Input: part model. Units: mm. Frame: model coordinates. A direction names the side the tool comes from. Coordinates: 2 decimals unless noted, no trailing zeros. Write each loop counter-clockwise with the first axis right and the second up, starting at its lowest first coordinate (ties: lowest second). Pieces come first, ordered by that corner, then holes. Notation, with made-up numbers: M 72,-38 L 83,-38 A8 cw 83,-26 Z; hole C -40,63 d10. An arc over 180 degrees is marked long. Write each question's results on one line, items separated by ' | '. Start each with the question number.
1. Set-up query: faces 1 (the flat face through (188, -110, 9)), 2 (the flat face through (104, -118, 11)). Return all of +Z, -Z, +X, -X, +Y, -Y with unobstructed straight access to the full face (end or side cutting, diameter ignored); none if empty.
2. First-contact query: pin 1 (5.5 mm diameter, centred on x = 80, y = -38, fed in from +Z); pin 2 (5 mm diameter, centred on x = 7, y = -6.5, fed in from +Z). Flat tips, straight axial feed; report the tip coordinate or a pass-through.
3. Section query B-B, the plane x = 88. Output: boundary loops of the cut face in (y, z).
4. Pull-direction query (X, two-part tool) for faces 3 (the flat face through (104, -58, 0)), 4 (the flat face through (8, -13, 9)), 5 (the flat face through (210, -60, 11)), 6 (the flat face through (8, -105, 9)); classes: +X half, -X half, draft (parallel to the pull), parting line (faces both ways), or undercut.
5. Section query A-A, the plane z = 5.5. Output: boundary loops of the cut face in (x, y), and give its area (3 significant figures).
6. Section query C-C, the plane y = -89. Output: boundary loops of the cut face in (x, z), and give its area (3 significant figures).
7. Ray query, probe 1 along X at (y, z) = (-110.5, 13); probe 2 along Y at (x, z) = (80, 1.95); probe 3 along X at (y, z) = (-13.5, 18.25). Return the intervals inside material, ascending.
```python
from build123d import *

# Parameters (mm, degrees)
F0_W     = 210
F0_H     = 118
F1_DEPTH = 23
F2_T     = -3
F3_W     = 10
F3_H     = 10
F4_DEPTH = 13
F5_R     = 1.75
F6_DEPTH = 25


with BuildPart() as f1:
    # F0 (on Top) → F1 (new body)
    with BuildSketch(Plane.XY):
        with Locations((105, -59)):
            Rectangle(F0_W, F0_H)
    extrude(amount=F1_DEPTH)

    # F2
    f2_openings = [f1.faces().sort_by_distance(p)[0] for p in [
        (105, -59, 23),
    ]]
    offset(amount=F2_T, openings=f2_openings)

    # F3 (on face) → F4 (join)
    with BuildSketch(Plane.XY.offset(3)):
        with Locations((8, -8)):
            Rectangle(F3_W, F3_H)
        with Locations((183, -8)):
            Rectangle(F3_W, F3_H)
        with Locations((183, -110)):
            Rectangle(F3_W, F3_H)
        with Locations((8, -110)):
            Rectangle(F3_W, F3_H)
    extrude(amount=F4_DEPTH)

    # F5 (on face) → F6 (cut)
    with BuildSketch(Plane.XY.offset(3)):
        with Locations((20, -8)):
            Circle(F5_R)
        with Locations((20, -38)):
            Circle(F5_R)
        with Locations((80, -38)):
            Circle(F5_R)
        with Locations((80, -8)):
            Circle(F5_R)
        with Locations((120, -17.5)):
            Circle(F5_R)
    extrude(amount=-F6_DEPTH, mode=Mode.SUBTRACT)


solid = f1.part
```
Answer:
1) face 1: +Z | face 2: +Z, -Z, +X, -X, -Y
2) pin 1: z = 3 | pin 2: z = 16
3) outline: M -118,0 L 0,0 L 0,23 L -3,23 L -3,3 L -115,3 L -115,23 L -118,23 Z
4) face 3: draft | face 4: undercut | face 5: +X half | face 6: undercut
5) outline: M 0,-118 L 210,-118 L 210,0 L 0,0 Z; hole M 3,-105 L 13,-105 L 13,-115 L 178,-115 L 178,-105 L 188,-105 L 188,-115 L 207,-115 L 207,-3 L 188,-3 L 188,-13 L 178,-13 L 178,-3 L 13,-3 L 13,-13 L 3,-13 Z | area: 2,330 mm^2
6) outline: M 0,0 L 210,0 L 210,23 L 207,23 L 207,3 L 3,3 L 3,23 L 0,23 Z | area: 750 mm^2
7) probe 1: 0 to 13, 178 to 188, 207 to 210 | probe 2: -118 to -39.75, -36.25 to -9.75, -6.25 to 0 | probe 3: 0 to 3, 207 to 210
